The model under review builds one solid part; all positions refer to its coordinate system, in mm. A direction names the side the tool comes from. Round coordinates to 2 decimals unless told otherwise and drop trailing zeros. Order: outer loops, then holes, each group sorted by start corner. A loop starts at its lowest first (then second) coordinate and runs counter-clockwise, first axis right, second up.
1) Mouldability with a two-part tool opening along X and no side actions: class faces 1 (the face through (43.825, 0.447, 7.776)), 2 (the face through (31.389, 23.244, 7.776)), 3 (the face through (11, -11, 40.234)) as pulls with the +X half, pulls with the -X half, needs draft (parallel to the pull), parting line crosses it, or undercut.
2) To check wall thickness, follow L1, parallel to X at y = -7, z = 4; L2, parallel to X at y = 2.5, z = 7; L3, parallel to Y at x = 0, z = 23.5. State the ranges of each line that lie inside material, in increasing order.
3) Clearance check with flat-ended pins moving along their axes: P1, Ø6, axis at x = 25.5, z = 7, coming from the +Y side; P2, Ø12, axis at y = -18.5, z = 28, coming from the +X side; P3, Ø10.5, axis at y = 0, z = 30, coming from the -X side; P4, Ø10, axis at x = 11, y = 21, coming from the -Z side. State where each tip first meets the part, or that it passes through.
4) Consider section A-A (z = 3.5). Give the number of separate pieces and of enclosed holes in the cut face, then the cut area to 3 significant figures.
5) Machinability: for faces 4 (the face through (22, 0, 0)), 5 (the face through (16, -4.9, 20)), which of the approach directions +Z, -Z, +X, -X, +Y, -Y give a long, thin tool a straight path to every point of the face, cutting with its end or side? Answer none if there is none.
6) Consider section B-B (z = 35). Give the boundary of the cut face in (x, y) (1 decimal).
from build123d import *

# Parameters (mm, degrees)
F1_DEPTH = 40.2336
F0_R     = 10.16
F2_DEPTH = 15.7734
F3_R     = 3.302


with BuildPart() as f1:
    # F0 (on Top) → F1 (new body)
    with BuildSketch(Plane.XY):
        with BuildLine():
            ThreePointArc((4.820397, -27.843313), (21.618264, -18.197169), (28.2575, 0))
            ThreePointArc((28.2575, 0), (21.618264, 18.197169), (4.820397, 27.843313))
            ThreePointArc((4.820397, 27.843313), (-28.2575, 0), (4.820397, -27.843313))
        make_face()
        with BuildLine():
            ThreePointArc((13.420816, -4.900444), (-14.287281, 0.079093), (13.474249, 4.751556))
            Line((13.474249, 4.751556), (18.5293, 4.751556))
            Line((18.5293, 4.751556), (18.5293, -4.900444))
            Line((18.5293, -4.900444), (13.420816, -4.900444))
        make_face(mode=Mode.SUBTRACT)
    extrude(amount=F1_DEPTH)

    # F0 (on Top) → F2 (join)
    with BuildSketch(Plane.XY):
        with BuildLine():
            ThreePointArc((4.820397, -27.843313), (21.618264, -18.197169), (28.2575, 0))
            ThreePointArc((28.2575, 0), (21.618264, 18.197169), (4.820397, 27.843313))
            ThreePointArc((4.820397, 27.843313), (-28.2575, 0), (4.820397, -27.843313))
        make_face()
        with BuildLine():
            ThreePointArc((13.420816, -4.900444), (-14.287281, 0.079093), (13.474249, 4.751556))
            Line((13.474249, 4.751556), (18.5293, 4.751556))
            Line((18.5293, 4.751556), (18.5293, -4.900444))
            Line((18.5293, -4.900444), (13.420816, -4.900444))
        make_face(mode=Mode.SUBTRACT)
        with BuildLine():
            ThreePointArc((4.820397, 27.843313), (21.618264, 18.197169), (28.2575, 0))
            ThreePointArc((28.2575, 0), (21.618264, -18.197169), (4.820397, -27.843313))
            Line((4.820397, -27.843313), (57.224706, -18.770773))
            ThreePointArc((57.224706, -18.770773), (73.025, 0), (57.224706, 18.770773))
            Line((57.224706, 18.770773), (4.820397, 27.843313))
        make_face()
        with Locations((53.975, 0)):
            Circle(F0_R, mode=Mode.SUBTRACT)
    extrude(amount=F2_DEPTH)

    # F3
    f3_edges = [f1.edges().sort_by_distance(p)[0] for p in [
        (-4.820397, 27.843313, 40.2336),
    ]]
    fillet(f3_edges, radius=F3_R)


solid = f1.part
Answer below:
1. face 1: undercut
1. face 2: pulls with the +X half
1. face 3: needs draft
2. L1: x = -27.38 to -12.46, 12.46 to 46.61, 61.34 to 71.69
2. L2: x = -28.15 to -14.07, 18.53 to 44.13, 63.82 to 72.86
2. L3: y = -28.26 to -14.29, 14.29 to 28.26
3. P1: stops at y = 24.78
3. P2: stops at x = 25.34
3. P3: stops at x = -28.26
3. P4: stops at z = 0
4. separate pieces: 1
4. enclosed holes: 2
4. area: 3,410 mm2
5. face 4: -Z, +X, -X, +Y, -Y
5. face 5: +Z, -Z
6. outline: circle Ø56.5 at (0, 0); hole (13.4, -4.9) - (18.5, -4.9) - (18.5, 4.8) - (13.5, 4.8) arc R14.3 ccw (long way) to start
